```python
from build123d import *

# Parameters (mm, degrees)
SKETCH1_W                = 806.45
SKETCH1_H                = 1981.2
BOSS_EXTRUDE1_DEPTH      = 3.175
SKETCH2_W                = 107.95
SKETCH2_H                = 965.2
SKETCH2_W_2              = 76.2
SKETCH2_H_2              = 101.6
CUT_EXTRUDE1_DEPTH       = 4.175
H_0_266_DIAMETER_HOLE1_D = 6.7564
SKETCH5_W                = 69.85
SKETCH5_H                = 76.2
CUT_EXTRUDE2_DEPTH       = 4.175
FILLET1_R                = 3.175
SKETCH7_R                = 17.399
CUT_EXTRUDE4_DEPTH       = 6.35
SKETCH8_W                = 44.45
SKETCH8_H                = 57.15
CUT_EXTRUDE5_DEPTH       = 4.175
SKETCH9_R                = 3.3782
CUT_EXTRUDE6_DEPTH       = 4.175
CUT_EXTRUDE7_DEPTH       = 4.175
CUT_EXTRUDE8_DEPTH       = 4.175
FILLET2_R                = 3.175


with BuildPart() as part:
    # Sketch1 → Boss-Extrude1 (new body)
    with BuildSketch(Plane(origin=(0, 0, 0), x_dir=(0, 0, -1), z_dir=(1, 0, 0))):
        with Locations((-403.225, 990.6)):
            Rectangle(SKETCH1_W, SKETCH1_H)
    extrude(amount=BOSS_EXTRUDE1_DEPTH)

    # Sketch2 → Cut-Extrude1 (cut, through all)
    with BuildSketch(Plane(origin=(3.175, 0, 0), x_dir=(0, 0, -1), z_dir=(1, 0, 0))):
        with Locations((-752.475, 482.6)):
            Rectangle(SKETCH2_W, SKETCH2_H)
        with Locations((-768.35, 1930.4)):
            Rectangle(SKETCH2_W_2, SKETCH2_H_2)
    extrude(amount=-CUT_EXTRUDE1_DEPTH, mode=Mode.SUBTRACT)

    # H (0.266) Diameter Hole1 (through all)
    with Locations(Plane(origin=(3.175, 0, 0), x_dir=(0, 0, -1), z_dir=(1, 0, 0))):
        with Locations((-50.00625, 1828.8), (-704.05625, 1828.8), (-648.49375, 1828.8), (-704.05625, 1493.52), (-648.49375, 1493.52), (-704.05625, 1158.24), (-648.49375, 1158.24), (-648.49375, 822.96), (-648.49375, 487.68), (-648.49375, 152.4), (-50.00625, 152.4), (-50.00625, 487.68), (-50.00625, 822.96), (-50.00625, 1158.24), (-50.00625, 1493.52), (-704.05625, 822.96), (-704.05625, 487.68), (-704.05625, 152.4)):
            Hole(H_0_266_DIAMETER_HOLE1_D / 2)

    # Sketch5 → Cut-Extrude2 (cut, through all)
    with BuildSketch(Plane(origin=(3.175, 0, 0), x_dir=(0, 0, -1), z_dir=(1, 0, 0))):
        with Locations((-117.475, 38.1)):
            Rectangle(SKETCH5_W, SKETCH5_H)
        with Locations((-581.025, 38.1)):
            Rectangle(SKETCH5_W, SKETCH5_H)
    extrude(amount=-CUT_EXTRUDE2_DEPTH, mode=Mode.SUBTRACT)

    # Fillet1
    fillet1_edges = [part.edges().sort_by_distance(p)[0] for p in [
        (1.5875, 76.2, 82.55),
        (1.5875, 0, 82.55),
        (1.5875, 0, 152.4),
        (1.5875, 76.2, 152.4),
        (1.5875, 76.2, 546.1),
        (1.5875, 0, 546.1),
        (1.5875, 0, 615.95),
        (1.5875, 76.2, 615.95),
        (1.5875, 965.2, 806.45),
        (1.5875, 965.2, 698.5),
        (1.5875, 0, 698.5),
        (1.5875, 1879.6, 806.45),
        (1.5875, 1981.2, 730.25),
        (1.5875, 1879.6, 730.25),
        (1.5875, 0, 0),
        (1.5875, 1981.2, 0),
    ]]
    fillet(fillet1_edges, radius=FILLET1_R)

    # Sketch7 → Cut-Extrude4 (cut)
    with BuildSketch(Plane(origin=(3.175, 0, 0), x_dir=(0, 0, -1), z_dir=(1, 0, 0))):
        with Locations((-285.75, 198.12)):
            Circle(SKETCH7_R)
    extrude(amount=-CUT_EXTRUDE4_DEPTH, mode=Mode.SUBTRACT)

    # Sketch8 → Cut-Extrude5 (cut, through all)
    with BuildSketch(Plane(origin=(3.175, 0, 0), x_dir=(0, 0, -1), z_dir=(1, 0, 0))):
        with Locations((-22.225, 263.525)):
            Rectangle(SKETCH8_W, SKETCH8_H)
    extrude(amount=-CUT_EXTRUDE5_DEPTH, mode=Mode.SUBTRACT)

    # Sketch9 → Cut-Extrude6 (cut, through all)
    with BuildSketch(Plane(origin=(3.175, 0, 0), x_dir=(0, 0, -1), z_dir=(1, 0, 0))):
        with Locations((-561.07957168, 1128.400068667)):
            Circle(SKETCH9_R)
        with Locations((-358.226152128, 975.539052786)):
            Circle(SKETCH9_R)
        with Locations((-155.372732576, 822.678036906)):
            Circle(SKETCH9_R)
    extrude(amount=-CUT_EXTRUDE6_DEPTH, mode=Mode.SUBTRACT)

    # Sketch10 → Cut-Extrude7 (cut, through all)
    with BuildSketch(Plane(origin=(3.175, 0, 0), x_dir=(0, 0, -1), z_dir=(1, 0, 0))):
        with BuildLine():
            Line((-44.45, 1282.7), (-44.45, 1028.7))
            ThreePointArc((-44.45, 1028.7), (-58.7375, 1014.4125), (-73.025, 1028.7))
            Line((-73.025, 1028.7), (-73.025, 1282.7))
            ThreePointArc((-73.025, 1282.7), (-58.7375, 1296.9875), (-44.45, 1282.7))
        make_face()
        with BuildLine():
            Line((-73.025, 1576.3875), (-73.025, 1611.3125))
            ThreePointArc((-73.025, 1611.3125), (-58.7375, 1625.6), (-44.45, 1611.3125))
            Line((-44.45, 1611.3125), (-44.45, 1576.3875))
            ThreePointArc((-44.45, 1576.3875), (-58.7375, 1562.1), (-73.025, 1576.3875))
        make_face()
        with BuildLine():
            Line((-44.45, 1928.8125), (-44.45, 1893.8875))
            ThreePointArc((-44.45, 1893.8875), (-58.7375, 1879.6), (-73.025, 1893.8875))
            Line((-73.025, 1893.8875), (-73.025, 1928.8125))
            ThreePointArc((-73.025, 1928.8125), (-58.7375, 1943.1), (-44.45, 1928.8125))
        make_face()
    extrude(amount=-CUT_EXTRUDE7_DEPTH, mode=Mode.SUBTRACT)

    # Sketch11 → Cut-Extrude8 (cut, through all)
    with BuildSketch(Plane(origin=(3.175, 0, 0), x_dir=(0, 0, -1), z_dir=(1, 0, 0))):
        with BuildLine():
            Line((-196.85, 736.6), (-196.85, 635))
            ThreePointArc((-196.85, 635), (-234.95, 596.9), (-273.05, 635))
            Line((-273.05, 635), (-273.05, 736.6))
            ThreePointArc((-273.05, 736.6), (-234.95, 774.7), (-196.85, 736.6))
        make_face()
        with BuildLine():
            Line((-196.85, 1346.2), (-196.85, 1193.8))
            ThreePointArc((-196.85, 1193.8), (-234.95, 1155.7), (-273.05, 1193.8))
            Line((-273.05, 1193.8), (-273.05, 1346.2))
            ThreePointArc((-273.05, 1346.2), (-234.95, 1384.3), (-196.85, 1346.2))
        make_face()
    extrude(amount=-CUT_EXTRUDE8_DEPTH, mode=Mode.SUBTRACT)

    # Fillet2
    fillet2_edges = [part.edges().sort_by_distance(p)[0] for p in [
        (1.5875, 292.1, 0),
        (1.5875, 234.95, 0),
        (1.5875, 234.95, 44.45),
        (1.5875, 292.1, 44.45),
    ]]
    fillet(fillet2_edges, radius=FILLET2_R)


solid = part.part
```
The listing builds one solid part. Answer for the finished solid, in the listing's coordinates (mm). A direction names the side the tool comes from. Round coordinates to 2 decimals unless told otherwise and drop trailing zeros. Loops run counter-clockwise (first coordinate to the right, second up) from the corner with the lowest first, then second, coordinate; pieces in that order, holes last. Notation, with made-up numbers: (37.25, 64) -> (73.25, 64) arc R23 ccw to (73.25, 79) -> close; hole circle Ø5 at (87.5, 53). An arc over 180 degrees is marked (long way). Use one line per item in the form item = value.
1. Find the intervals of material crossed by probe 1 along Z at (x, y) = (1.1, 1828.8); probe 2 along Z at (x, y) = (1.5, 727); probe 3 along Y at (x, z) = (2.2, 203), in increasing order. Write a range as [from, to].
Answer key:
probe_1 = [0, 46.63], [53.38, 645.12], [651.87, 700.68], [707.43, 806.45]
probe_2 = [0, 196.85], [273.05, 698.5]
probe_3 = [0, 614.24], [757.36, 1173.04], [1366.96, 1981.2]
2. The part is cut by section A-A on y = 198.12. Determine the outline of the cut face in (x, z) (3 decimals).
Answer key:
outline = (0, 0) -> (3.175, 0) -> (3.175, 268.351) -> (0, 268.351) -> close; (0, 303.149) -> (3.175, 303.149) -> (3.175, 698.5) -> (0, 698.5) -> close
3. Flat-ended cylindrical pins translate along their axes: pin 1 Ø5.5 at (y, z) = (487.68, 50.01) entering from -X; pin 2 Ø1.6 at (x, y) = (2, 274) entering from -Z. Find the tip coordinate at first contact, or state that the pin passes through.
Answer key:
pin_1 = through
pin_2 = 44.45
4. For a pull along Y with two mould halves and no side action, classify faces 3 (the flat face through (3.175, 1004, 409)), 4 (the cylindrical face through (1.61, 215.37, 288.02)) as released by +Y, released by -Y, zero draft, split by the parting line, or undercut.
Answer key:
face_3 = zero draft
face_4 = undercut
5. A tool of negligible diameter and unlimited length cuts with its end or side. For faces 1 (the flat face through (0, 1004, 409)), 2 (the cylindrical face through (1.61, 1384.29, 235.79)), from which of +Z, -Z, +X, -X, +Y, -Y can it reach the whole face along a straight path? Write none if from no direction.
Answer key:
face_1 = +Z, -Z, -X, +Y, -Y
face_2 = +X, -X
6. The part is cut by section C-C on y = 800. Determine the outline of the cut face in (x, z) (3 decimals), and give its area (3 significant figures).
Answer key:
outline = (0, 0) -> (3.175, 0) -> (3.175, 698.5) -> (0, 698.5) -> close
area = 2,220 mm²
7. The part is cut by section B-B on x = 2.35. Give the number of separate pieces and of enclosed holes in the cut face, and give its area (3 significant figures).
Answer key:
separate_pieces = 1
enclosed_holes = 23
area = 1,430,000 mm²
